Design review of the part built by this model. Coordinates are the model's own, in mm. A direction names the side the tool comes from. Give positions to 0.01 mm unless a question says otherwise; leave off trailing zeros. Write each loop counter-clockwise with the first axis right and the second up, starting at its lowest first coordinate (ties: lowest second). Pieces come first, ordered by that corner, then holes. Notation, with made-up numbers: M 4,85.5 L 18,85.5 A32 cw 18,118.5 Z; hole C 66,20.25 d2. An arc over 180 degrees is marked long. Use a Markdown table: item, result. Add a question column.
```python
from build123d import *

# Parameters (mm, degrees)
F0_R     = 25.4
F1_DEPTH = 12.7
F2_R     = 2.54
F3_DEPTH = 12.7
F4_R     = 3.2385
F5_DEPTH = 12.7


with BuildPart() as f1:
    # F0 (on Front) → F1 (new body)
    with BuildSketch(Plane.XZ):
        Circle(F0_R)
    extrude(amount=F1_DEPTH)

    # F2 (on face) → F3 (join)
    with BuildSketch(Plane(origin=(0, 0, 0), x_dir=(-1, 0, 0), z_dir=(0, 1, 0))):
        with Locations((12.313798, 15.931344)):
            Circle(F2_R)
        with Locations((0.597863, 20.126597)):
            Circle(F2_R)
        with Locations((-11.346435, 16.634174)):
            Circle(F2_R)
        with Locations((-18.956781, 6.788062)):
            Circle(F2_R)
        with Locations((-19.326281, -5.650859)):
            Circle(F2_R)
        with Locations((-12.313798, -15.931344)):
            Circle(F2_R)
        with Locations((-0.597863, -20.126597)):
            Circle(F2_R)
        with Locations((11.346435, -16.634174)):
            Circle(F2_R)
        with Locations((18.956781, -6.788062)):
            Circle(F2_R)
        with Locations((19.326281, 5.650859)):
            Circle(F2_R)
    extrude(amount=F3_DEPTH)

    # F4 (on face) → F5 (cut)
    with BuildSketch(Plane(origin=(0, 0, 0), x_dir=(-1, 0, 0), z_dir=(0, 1, 0))):
        Circle(F4_R)
    extrude(amount=-F5_DEPTH, mode=Mode.SUBTRACT)


solid = f1.part
```
(1) Add section D-D on x = -12. Give the boundary of the cut face in (y, z).
(2) Add section C-C on x = 0. Give the boundary of the cut face in (y, z).
(3) Wall thickness on L1, parallel to Z at x = 0, y = -7.5; L2, parallel to Y at x = 16.5, z = 14; L3, parallel to Z at x = -18, y = 7.75: over which ranges is each line inside the solid? List them lowest first.
(4) Add section A-A on z = 0. Give the boundary of the cut face in (x, y), then the cut area to 3 significant figures.
(5) Add section B-B on y = 0.75. Give the number of separate pieces and of enclosed holes in the cut face, then the cut area to 3 significant figures.
(6) For pin 1 (3 mm diameter, centred on x = -5.5, y = -7, fed in from +Z); pin 2 (2 mm diameter, centred on x = 17, y = -2, fed in from -Z); pin 3 (3 mm diameter, centred on x = 13, z = -3.5, fed in from +Y), all flat-tipped, find the tip position at first contact; note any pin that passes through.
(7) Machinability: for faces 4 (the flat face through (5, 0, 0)), 5 (the flat face through (19, 12.7, -6)), which of the approach directions +Z, -Z, +X, -X, +Y, -Y give a long, thin tool a straight path to every point of the face, cutting with its end or side? Answer none if there is none.
(8) The part is to be moulded in two halves that separate along X. For faces 1 (the flat face through (12, 12.7, -16)), 2 (the cylindrical face through (-5.506, -6.261, -24.796)), 3 (the cylindrical face through (21.494, 6.261, 6.9)), say which applies: released by +X, released by -X, zero draft, split by the parting line, or undercut.
From the geometry:
| question | item | result |
|---|---|---|
| 1 | outline | M -12.7,-22.39 L 0,-22.39 L 0,-19.09 L 12.7,-19.09 L 12.7,-14.18 L 0,-14.18 L 0,13.41 L 12.7,13.41 L 12.7,18.45 L 0,18.45 L 0,22.39 L -12.7,22.39 Z |
| 2 | outline | M -12.7,-25.4 L 0,-25.4 L 0,-22.6 L 12.7,-22.6 L 12.7,-17.66 L 0,-17.66 L 0,-3.24 L -12.7,-3.24 Z; M -12.7,3.24 L 0,3.24 L 0,17.66 L 12.7,17.66 L 12.7,22.6 L 0,22.6 L 0,25.4 L -12.7,25.4 Z |
| 3 | L1 | z = -25.4 to -3.24, 3.24 to 25.4 |
| 3 | L2 | y = -12.7 to 0 |
| 3 | L3 | z = -9.14 to -4.44, 3.48 to 7.82 |
| 4 | outline | M -25.4,-12.7 L -3.24,-12.7 L -3.24,0 L -25.4,0 Z; M 3.24,-12.7 L 25.4,-12.7 L 25.4,0 L 3.24,0 Z |
| 4 | area | 563 mm^2 |
| 5 | separate pieces | 10 |
| 5 | enclosed holes | 0 |
| 5 | area | 203 mm^2 |
| 6 | pin 1 | stops at z = 25.08 |
| 6 | pin 2 | stops at z = -19.73 |
| 6 | pin 3 | stops at y = 0 |
| 7 | face 4 | +Y |
| 7 | face 5 | +Z, -Z, +X, -X, +Y |
| 8 | face 1 | zero draft |
| 8 | face 2 | split by the parting line |
| 8 | face 3 | undercut |
